Read the model definition and answer for the solid it produces. Units are mm, in the model's axes. Face numbers are marked on the shaded views. A direction names the side the tool comes from. Give positions to 0.01 mm unless a question says otherwise; leave off trailing zeros. Write each loop counter-clockwise with the first axis right and the second up, starting at its lowest first coordinate (ties: lowest second). Pieces come first, ordered by that corner, then holes. Notation, with made-up numbers: (25, 30.25) -> (44, 30.25) arc R28 ccw to (44, 56.25) -> close; hole circle Ø9 at (24.25, 64). An arc over 180 degrees is marked (long way). Use a Markdown table: item, result.
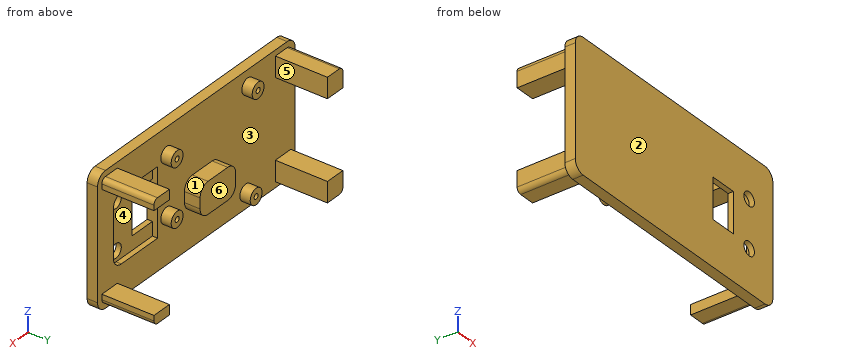
from build123d import *

# Parameters (mm, degrees)
SKETCH1_W            = 127
SKETCH1_H            = 63.5
BOSS_EXTRUDE1_DEPTH  = 5.08
SKETCH2_W            = 9.906
SKETCH2_H            = 9.906
SKETCH2_H_2          = 4.826
BOSS_EXTRUDE3_DEPTH  = 25.4
FILLET3_R            = 2.286
FILLET4_R            = 5.08
CUT_EXTRUDE8_REACH   = 146.244
SKETCH13_R           = 3.556
SKETCH13_W           = 13.208
SKETCH13_H           = 19.558
SKETCH14_W           = 13.208
SKETCH14_H           = 29.718
CUT_EXTRUDE9_DEPTH   = 2.54
SKETCH19_R           = 5.08
CUT_EXTRUDE12_DEPTH  = 2.54
SKETCH4_R            = 3.81
SKETCH4_R_2          = 1.27
BOSS_EXTRUDE13_DEPTH = 5.08
SKETCH7_W            = 22.86
SKETCH7_H            = 15.24
BOSS_EXTRUDE14_DEPTH = 7.62
FILLET5_R            = 5.08
CUT_EXTRUDE13_DEPTH  = 2.54
SKETCH22_R           = 4.329078616
SKETCH22_R_2         = 3.3655
SKETCH22_R_3         = 4.536345421
BOSS_EXTRUDE15_DEPTH = 2.54


with BuildPart() as part:
    # Sketch1 → Boss-Extrude1 (new body)
    with BuildSketch(Plane(origin=(0, 0, 0), x_dir=(1, 0, 0), z_dir=(0, 1, 0))):
        with Locations((63.5, 31.75)):
            Rectangle(SKETCH1_W, SKETCH1_H)
    extrude(amount=BOSS_EXTRUDE1_DEPTH)

    # Sketch2 → Boss-Extrude3 (add)
    with BuildSketch(Plane(origin=(0, 5.08, 0), x_dir=(1, 0, 0), z_dir=(0, 1, 0))):
        with Locations((7.747, 7.747)):
            Rectangle(SKETCH2_W, SKETCH2_H)
        with Locations((7.747, 55.753)):
            Rectangle(SKETCH2_W, SKETCH2_H)
        with Locations((119.253, 5.207)):
            Rectangle(SKETCH2_W, SKETCH2_H_2)
        with Locations((119.253, 58.293)):
            Rectangle(SKETCH2_W, SKETCH2_H_2)
    extrude(amount=BOSS_EXTRUDE3_DEPTH)

    # Fillet3
    fillet3_edges = [part.edges().sort_by_distance(p)[0] for p in [
        (2.794, 17.78, -60.706),
        (2.794, 17.78, -2.794),
        (124.206, 17.78, -60.706),
        (124.206, 17.78, -2.794),
    ]]
    fillet(fillet3_edges, radius=FILLET3_R)

    # Fillet4
    fillet4_edges = [part.edges().sort_by_distance(p)[0] for p in [
        (0, 2.54, -63.5),
        (127, 2.54, -63.5),
        (127, 2.54, 0),
        (0, 2.54, 0),
    ]]
    fillet(fillet4_edges, radius=FILLET4_R)

    # Sketch13 → Cut-Extrude8 (cut, up to next)
    with BuildSketch(Plane(origin=(0, 5.08, 0), x_dir=(1, 0, 0), z_dir=(0, 1, 0)), mode=Mode.PRIVATE) as cut_extrude8_sk1:
        with Locations(Location((111.76, 43.18, 0), (0, 0, 270))):
            Circle(SKETCH13_R)
    cut_extrude8_tool1 = extrude(cut_extrude8_sk1.sketch, amount=-CUT_EXTRUDE8_REACH, mode=Mode.PRIVATE) & part.part
    # Sketch13 → Cut-Extrude8 (cut, up to next)
    with BuildSketch(Plane(origin=(0, 5.08, 0), x_dir=(1, 0, 0), z_dir=(0, 1, 0)), mode=Mode.PRIVATE) as cut_extrude8_sk2:
        with Locations(Location((111.76, 20.32, 0), (0, 0, 270))):
            Circle(SKETCH13_R)
    cut_extrude8_tool2 = extrude(cut_extrude8_sk2.sketch, amount=-CUT_EXTRUDE8_REACH, mode=Mode.PRIVATE) & part.part
    # Sketch13 → Cut-Extrude8 (cut, up to next)
    with BuildSketch(Plane(origin=(0, 5.08, 0), x_dir=(1, 0, 0), z_dir=(0, 1, 0)), mode=Mode.PRIVATE) as cut_extrude8_sk3:
        with Locations((94.996, 31.75)):
            Rectangle(SKETCH13_W, SKETCH13_H)
    cut_extrude8_tool3 = extrude(cut_extrude8_sk3.sketch, amount=-CUT_EXTRUDE8_REACH, mode=Mode.PRIVATE) & part.part
    add(cut_extrude8_tool1.solids().sort_by_distance((111.76, 5.08, -43.18))[0], mode=Mode.SUBTRACT)
    add(cut_extrude8_tool2.solids().sort_by_distance((111.76, 5.08, -20.32))[0], mode=Mode.SUBTRACT)
    add(cut_extrude8_tool3.solids().sort_by_distance((94.996, 5.08, -31.75))[0], mode=Mode.SUBTRACT)

    # Sketch14 → Cut-Extrude9 (cut)
    with BuildSketch(Plane(origin=(0, 5.08, 0), x_dir=(1, 0, 0), z_dir=(0, 1, 0))):
        with Locations((94.996, 31.75)):
            Rectangle(SKETCH14_W, SKETCH14_H)
    extrude(amount=-CUT_EXTRUDE9_DEPTH, mode=Mode.SUBTRACT)

    # Sketch19 → Cut-Extrude12 (cut)
    with BuildSketch(Plane(origin=(0, 5.08, 0), x_dir=(1, 0, 0), z_dir=(0, 1, 0))):
        with Locations(Location((111.76, 43.18, 0), (0, 0, 270))):
            Circle(SKETCH19_R)
        with Locations(Location((111.76, 20.32, 0), (0, 0, 270))):
            Circle(SKETCH19_R)
    extrude(amount=-CUT_EXTRUDE12_DEPTH, mode=Mode.SUBTRACT)

    # Sketch4 → Boss-Extrude13 (add)
    # profile 1 of 4: a face of its own
    with BuildSketch(Plane(origin=(0, 5.08, 0), x_dir=(1, 0, 0), z_dir=(0, 1, 0))):
        with Locations(Location((31.75, 55.88, 0), (0, 0, 90))):
            Circle(SKETCH4_R)
        with Locations(Location((31.75, 55.88, 0), (0, 0, 270))):
            Circle(SKETCH4_R_2, mode=Mode.SUBTRACT)
    # profile 2 of 4: a face of its own
    with BuildSketch(Plane(origin=(0, 5.08, 0), x_dir=(1, 0, 0), z_dir=(0, 1, 0))):
        with Locations(Location((30.48, 7.62, 0), (0, 0, 90))):
            Circle(SKETCH4_R)
        with Locations(Location((30.48, 7.62, 0), (0, 0, 270))):
            Circle(SKETCH4_R_2, mode=Mode.SUBTRACT)
    # profile 3 of 4: a face of its own
    with BuildSketch(Plane(origin=(0, 5.08, 0), x_dir=(1, 0, 0), z_dir=(0, 1, 0))):
        with Locations(Location((82.55, 40.64, 0), (0, 0, 90))):
            Circle(SKETCH4_R)
        with Locations(Location((82.55, 40.64, 0), (0, 0, 270))):
            Circle(SKETCH4_R_2, mode=Mode.SUBTRACT)
    # profile 4 of 4: a face of its own
    with BuildSketch(Plane(origin=(0, 5.08, 0), x_dir=(1, 0, 0), z_dir=(0, 1, 0))):
        with Locations(Location((82.55, 12.7, 0), (0, 0, 90))):
            Circle(SKETCH4_R)
        with Locations(Location((82.55, 12.7, 0), (0, 0, 270))):
            Circle(SKETCH4_R_2, mode=Mode.SUBTRACT)
    extrude(amount=BOSS_EXTRUDE13_DEPTH)

    # Sketch7 → Boss-Extrude14 (add)
    with BuildSketch(Plane(origin=(0, 5.08, 0), x_dir=(1, 0, 0), z_dir=(0, 1, 0))):
        with Locations((59.69, 38.1)):
            Rectangle(SKETCH7_W, SKETCH7_H)
    extrude(amount=BOSS_EXTRUDE14_DEPTH)

    # Fillet5
    fillet5_edges = [part.edges().sort_by_distance(p)[0] for p in [
        (48.26, 8.89, -45.72),
        (48.26, 8.89, -30.48),
        (71.12, 8.89, -30.48),
        (71.12, 8.89, -45.72),
    ]]
    fillet(fillet5_edges, radius=FILLET5_R)

    # Sketch21 → Cut-Extrude13 (cut)
    with BuildSketch(Plane(origin=(0, 5.08, 0), x_dir=(1, 0, 0), z_dir=(0, 1, 0))):
        with BuildLine():
            Line((111.76, 48.26), (88.392, 48.26))
            Line((88.392, 48.26), (88.392, 15.24))
            Line((88.392, 15.24), (111.76, 15.24))
            ThreePointArc((111.76, 15.24), (115.352102448, 16.727897552), (116.84, 20.32))
            Line((116.84, 20.32), (116.84, 43.18))
            ThreePointArc((116.84, 43.18), (115.352102448, 46.772102448), (111.76, 48.26))
        make_face()
    extrude(amount=-CUT_EXTRUDE13_DEPTH, mode=Mode.SUBTRACT)

    # Sketch22 → Boss-Extrude15 (add)
    # profile 1 of 2: a face of its own
    with BuildSketch(Plane(origin=(0, 2.54, 0), x_dir=(1, 0, 0), z_dir=(0, 1, 0))):
        with Locations((111.76, 43.18)):
            Circle(SKETCH22_R)
        with Locations(Location((111.76, 43.18, 0), (0, 0, 270))):
            Circle(SKETCH22_R_2, mode=Mode.SUBTRACT)
    # profile 2 of 2: a face of its own
    with BuildSketch(Plane(origin=(0, 2.54, 0), x_dir=(1, 0, 0), z_dir=(0, 1, 0))):
        with Locations((111.76, 20.32)):
            Circle(SKETCH22_R_3)
        with Locations(Location((111.76, 20.32, 0), (0, 0, 270))):
            Circle(SKETCH22_R_2, mode=Mode.SUBTRACT)
    extrude(amount=-BOSS_EXTRUDE15_DEPTH)


solid = part.part
Item 1: A cutting plane is placed at D-D (x = 24.5). Give the vertices of the cut face in (y, z), then the cut area to 3 significant figures.
Return value:
| item | result |
|---|---|
| outline | (0, -63.5) -> (5.08, -63.5) -> (5.08, 0) -> (0, 0) -> close |
| area | 323 mm^2 |
Item 2: For a pull along Z with two mould halves and no side action, classify the marked faces 1, 2 and 3 as +Z half, -Z half, draft (parallel to the pull), parting line (faces both ways), or undercut.
Return value:
| item | result |
|---|---|
| face 1 | +Z half |
| face 2 | draft |
| face 3 | undercut |
Item 3: A cutting plane is placed at C-C (x = 68). Give the vertices of the cut face in (y, z).
Return value:
| item | result |
|---|---|
| outline | (0, -63.5) -> (5.08, -63.5) -> (5.08, -45.33) -> (12.7, -45.33) -> (12.7, -30.87) -> (5.08, -30.87) -> (5.08, 0) -> (0, 0) -> close |
Item 4: Each of these flat-tipped pins is pushed along its axis until it touches: P1, Ø4, axis at y = 14, z = -4.5, coming from the -X side; P2, Ø4, axis at x = 111.76, z = -20.32, coming from the -Y side; P3, Ø8.5, axis at x = 84, z = -39.5, coming from the +Y side; P4, Ø1.3, axis at x = 30.5, z = -7.5, coming from the +Y side. Where does it stop, or does it pass through?
Return value:
| item | result |
|---|---|
| P1 | x = 2.79 |
| P2 | through |
| P3 | y = 10.16 |
| P4 | y = 5.08 |
Item 5: A cutting plane is placed at A-A (y = 15.5). Give the vertices of the cut face in (x, z).
Return value:
| item | result |
|---|---|
| outline | (2.79, -58.42) arc R2.29 ccw to (5.08, -60.71) -> (12.7, -60.71) -> (12.7, -50.8) -> (2.79, -50.8) -> close; (2.79, -12.7) -> (12.7, -12.7) -> (12.7, -2.79) -> (5.08, -2.79) arc R2.29 ccw to (2.79, -5.08) -> close; (114.3, -60.71) -> (121.92, -60.71) arc R2.29 ccw to (124.21, -58.42) -> (124.21, -55.88) -> (114.3, -55.88) -> close; (114.3, -7.62) -> (124.21, -7.62) -> (124.21, -5.08) arc R2.29 ccw to (121.92, -2.79) -> (114.3, -2.79) -> close |
Item 6: Straight lines are drawn through the part: line 1 along X through (y, z) = (1.75, -20.32); line 2 along X through (y, z) = (7, -55); line 3 along Z through (x, y) = (8.5, 9.5). For each, find the intervals that lie inside material, in ascending order. Write a range as [from, to].
Return value:
| item | result |
|---|---|
| line 1 | [0, 108.39], [115.13, 127] |
| line 2 | [2.79, 12.7], [28.04, 30.83], [32.67, 35.46] |
| line 3 | [-60.71, -50.8], [-12.7, -2.79] |
Item 7: A tool of negligible diameter and unlimited length cuts with its end or side. For the marked faces 4, 5 and 6, from which of +Z, -Z, +X, -X, +Y, -Y can it reach the whole face along a straight path? Write none if from no direction.
Return value:
| item | result |
|---|---|
| face 4 | +Y |
| face 5 | +Z, -Z, +Y |
| face 6 | +Z, -Z, +X, -X, +Y |
Item 8: A cutting plane is placed at B-B (x = 82.55). Give the vertices of the cut face in (y, z).
Return value:
| item | result |
|---|---|
| outline | (0, -63.5) -> (5.08, -63.5) -> (5.08, -44.45) -> (10.16, -44.45) -> (10.16, -41.91) -> (5.08, -41.91) -> (5.08, -39.37) -> (10.16, -39.37) -> (10.16, -36.83) -> (5.08, -36.83) -> (5.08, -16.51) -> (10.16, -16.51) -> (10.16, -13.97) -> (5.08, -13.97) -> (5.08, -11.43) -> (10.16, -11.43) -> (10.16, -8.89) -> (5.08, -8.89) -> (5.08, 0) -> (0, 0) -> close |
